Can you work these out from the model? Positions are in its coordinate system, mm. Face numbers are marked on the shaded views. A direction names the side the tool comes from. Give positions to 0.01 mm unless a question says otherwise; leave off trailing zeros. Loops run counter-clockwise (first coordinate to the right, second up) from the corner with the lowest first, then second, coordinate; pieces in that order, holes last. Notation, with made-up numbers: M 17.5,81.5 L 26.5,81.5 A34 ccw 26.5,119.5 Z; hole C 52,49.5 d5. An arc over 180 degrees is marked long. Use CSV: the item, a comma, the result in double quotes.
from build123d import *

# Parameters (mm, degrees)
SKETCH2_OUTSIDE_W   = 21.592
SKETCH2_OUTSIDE_H   = 21.592
SKETCH2_OUTSIDE_W_2 = 21.785609725
SKETCH2_OUTSIDE_H_2 = 12
CUT_EXTRUDE1_DEPTH  = 21


with BuildPart() as part:
    # Sketch1 → Revolve1 (revolve)
    with BuildSketch(Plane.XY):
        Polygon((5.1435, -5.969), (1.5875, -5.969), (1.5875, -17.90602957), (0.25, -19.5), (0.25, -20), (4.722297129, -16.247297129), (4.5, -16.025), (5, -15.525), (4.5, -15.025), (5, -14.525), (4.5, -14.025), (5, -13.525), (4.5, -13.025), (5, -12.525), (4.5, -12.025), (5, -11.525), (4.5, -11.025), (5, -10.525), (4.5, -10.025), (5, -9.525), (4.5, -9.525), (4.5, -8.001), (6.985, -8.001), (6.985, 0), (4.555, 0), (5, -0.445), (4.5, -0.945), (5, -1.445), (4.5, -1.945), (5, -2.445), (4.5, -2.945), (5, -3.445), (4.5, -3.945), (5, -4.445), (5.1435, -4.445), align=None)
    revolve(axis=Axis((0, 0, 0), (0, -1, 0)))

    # Sketch2 outside → Cut-Extrude1 (cut, through all)
    with BuildSketch(Plane(origin=(0, 0, 0), x_dir=(1, 0, 0), z_dir=(0, 1, 0))):
        Rectangle(SKETCH2_OUTSIDE_W, SKETCH2_OUTSIDE_H)
        with Locations((0.61693762, 0)):
            Rectangle(SKETCH2_OUTSIDE_W_2, SKETCH2_OUTSIDE_H_2, mode=Mode.SUBTRACT)
    extrude(amount=-CUT_EXTRUDE1_DEPTH, mode=Mode.SUBTRACT)


solid = part.part
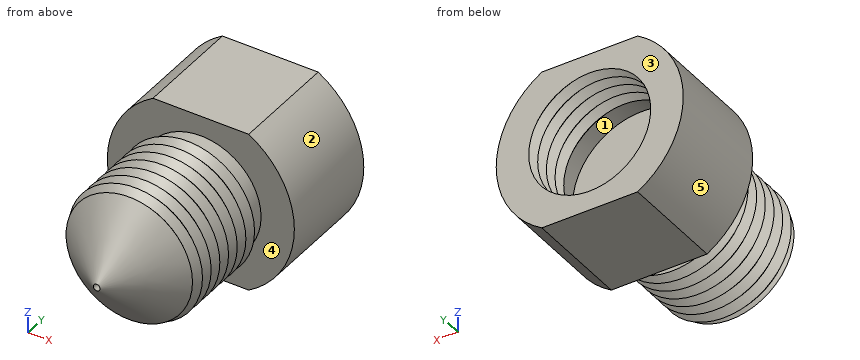
Q1. I want a section at A-A, the plane x = 6. Please give me the cut outline in (y, z), then the cut area to 3 significant figures.
Model answer:
outline,"M -8,-3.58 L 0,-3.58 L 0,3.58 L -8,3.58 Z"
area,"57.2 mm2"
Q2. For the marked faces 4 and 5, which set-ups out of +Z, -Z, +X, -X, +Y, -Y let a thin tool reach every point of the face, with its end or its side?
Model answer:
face 4,"none"
face 5,"-X, +Y, -Y"
Q3. Please list where these lines run through material, in increasing order: L1, parallel to Z at x = 0, y = -4.9; L2, parallel to Y at x = -1.25, z = 5.75; L3, parallel to Z at x = 0, y = -12.75 (1 decimal). Write a range as from..to.
Model answer:
L1,"-6..-5.14, 5.14..6"
L2,"-8..0"
L3,"-4.8..-1.6, 1.6..4.8"
Q4. I want a section at B-B, the plane x = -5.5. Please give me the cut outline in (y, z).
Model answer:
outline,"M -8,-4.31 L 0,-4.31 L 0,4.31 L -8,4.31 Z"
Q5. If we mould it in two halves opening along X, with no side actions, what happens to the marked faces 1, 2 and 3? For each: released by +X, released by -X, zero draft, split by the parting line, or undercut.
Model answer:
face 1,"undercut"
face 2,"released by +X"
face 3,"zero draft"
Q6. I'm going to push flat-ended pins straight in: P1, Ø3, axis at x = 2, z = -1, coming from the -Y side; P2, Ø1.5, axis at x = -3.5, y = -11.5, coming from the -Z side; P3, Ø2.5, axis at x = 0, z = 0, coming from the +Y side. Where does each tip first touch, or does it pass through?
Model answer:
P1,"y = -19.59"
P2,"z = -4.18"
P3,"y = -18.31"
